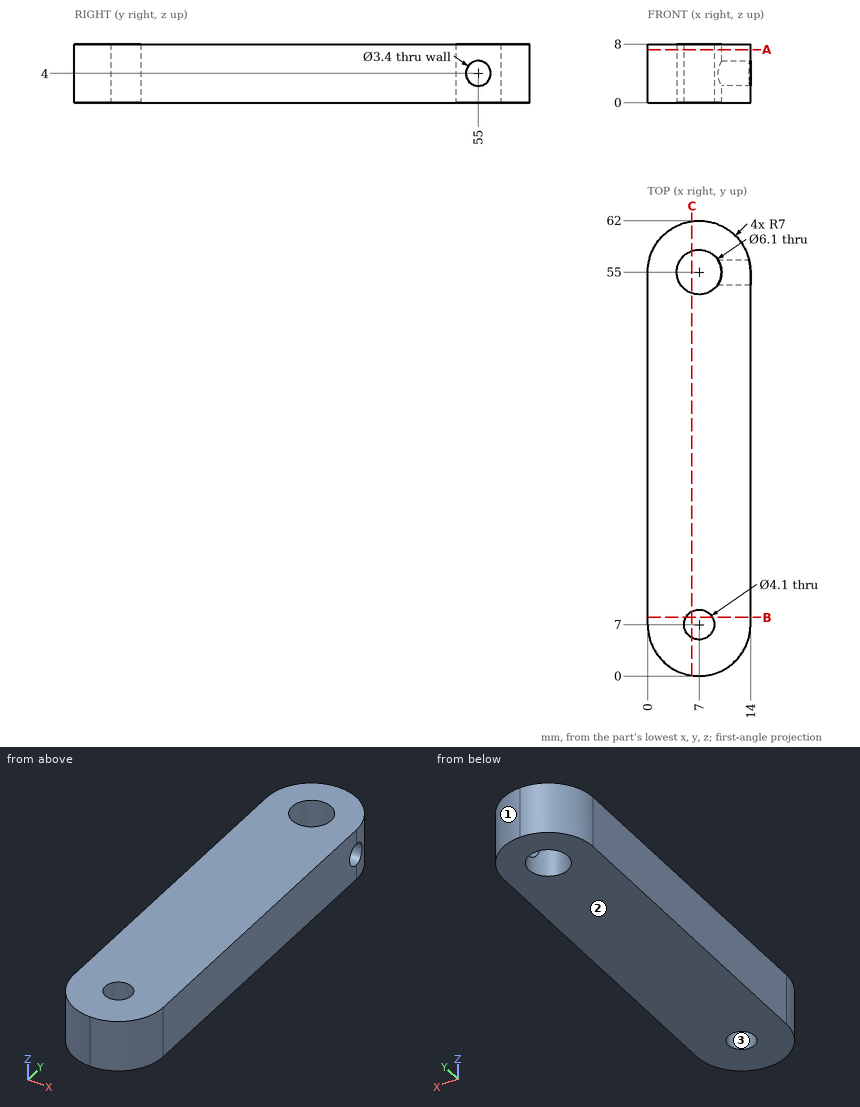
Drawing for the job (mm, zero at the part's lowest x, y, z). Round coordinates to 2 decimals unless told otherwise and drop trailing zeros. Loops run counter-clockwise (first coordinate to the right, second up) from the corner with the lowest first, then second, coordinate; pieces in that order, holes last. Notation, with made-up numbers: (47, -31.5) -> (95, -31.5) arc R25 ccw to (95, -12.5) -> close; hole circle Ø10 at (30, 15). An arc over 180 degrees is marked (long way). Answer in a Markdown table with one row per item.
Item 1: Pin check, flat tips, straight feed: pin 1 (3 mm diameter, centred on x = 10.5, z = 3, fed in from -Y); pin 2 (1.5 mm diameter, centred on x = 3.5, z = 6.5, fed in from +Y). Stop position of each tip, or through.
Answers below:
| item | result |
|---|---|
| pin 1 | stops at y = 0.29 |
| pin 2 | stops at y = 61.44 |
Item 2: Saw through at C-C (x = 6). Write the cut outline in (y, z).
Answers below:
| item | result |
|---|---|
| outline | (0.07, 0) -> (5.21, 0) -> (5.21, 8) -> (0.07, 8) -> close; (8.79, 0) -> (52.12, 0) -> (52.12, 8) -> (8.79, 8) -> close; (57.88, 0) -> (61.93, 0) -> (61.93, 8) -> (57.88, 8) -> close |
Item 3: Saw through at B-B (y = 8). Write the cut outline in (x, z).
Answers below:
| item | result |
|---|---|
| outline | (0, 0) -> (5.21, 0) -> (5.21, 8) -> (0, 8) -> close; (8.79, 0) -> (14, 0) -> (14, 8) -> (8.79, 8) -> close |
Item 4: Mould opens along X. For the marked faces 1, 2 and 3 say: +X half, -X half, draft (parallel to the pull), parting line (faces both ways), or undercut.
Answers below:
| item | result |
|---|---|
| face 1 | +X half |
| face 2 | draft |
| face 3 | undercut |
Item 5: Drill centre lines: L1, parallel to Y at x = 7, z = 5; L2, parallel to X at y = 55, z = 4.25; L3, parallel to Z at x = 12.5, y = 55. Where is each one in solid material? Low to high. Write a range as [from, to].
Answers below:
| item | result |
|---|---|
| L1 | y = [0, 4.95], [9.05, 51.95], [58.05, 62] |
| L2 | x = [0, 3.95] |
| L3 | z = [0, 2.3], [5.7, 8] |
Item 6: Saw through at A-A (z = 7.25). State how many separate pieces and enclosed holes the cut face has, and give its area (4 significant figures).
Answers below:
| item | result |
|---|---|
| separate pieces | 1 |
| enclosed holes | 2 |
| area | 783.5 mm² |
